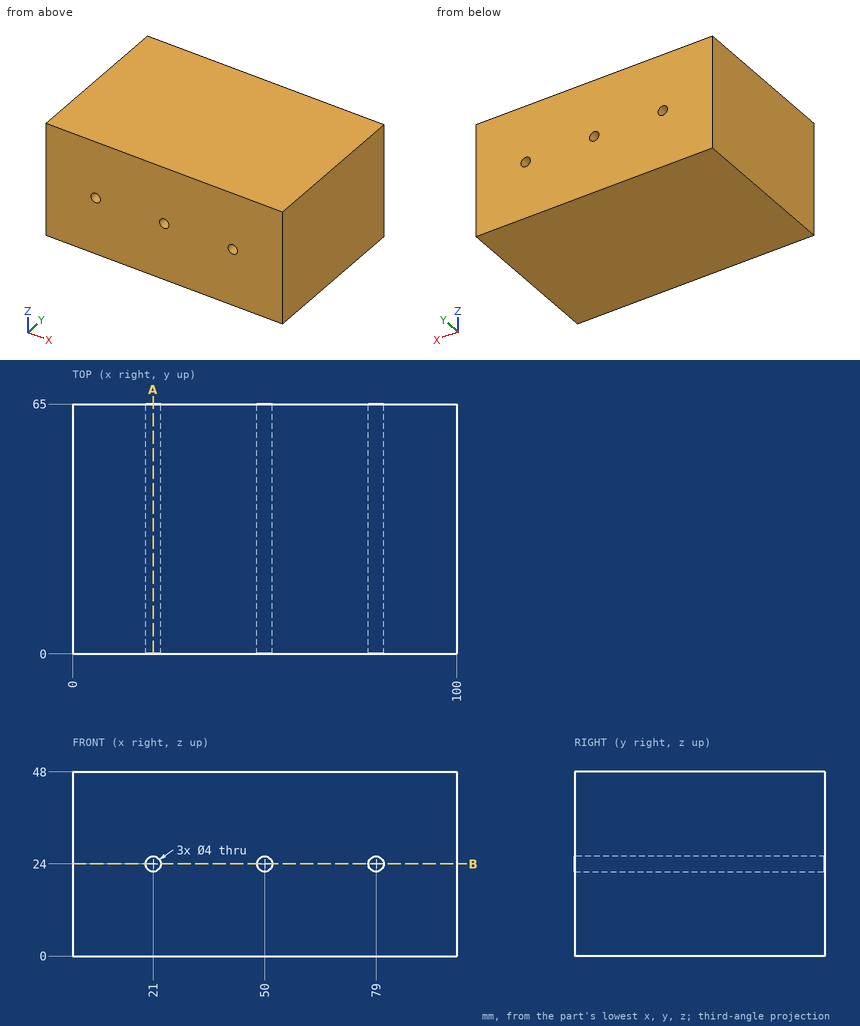
Check sheet for the drawn part. Datum: minimum x, y, z corner. Units: mm. Round coordinates to 2 decimals unless told otherwise and drop trailing zeros. Write each loop counter-clockwise with the first axis right and the second up, starting at its lowest first coordinate (ties: lowest second). Pieces come first, ordered by that corner, then holes. Notation, with made-up numbers: (7, 74.5) -> (61, 74.5) arc R19 ccw to (61, 101.5) -> close; hole circle Ø1 at (89, 67.25). An arc over 180 degrees is marked (long way). Write each question's results on one line, items separated by ' | '. Start each with the question number.
1. Cross-section at A-A (x = 21). Enter the section's corners in (y, z).
2. Depth check by flat-ended pin: P1, Ø10, axis at x = 60, y = 7, coming from the -Z side. Enter the tip coordinate at first touch or a pass-through.
3. Material ranges on probe 1 along X at (y, z) = (30, 24); probe 2 along Z at (x, y) = (79, 47); probe 3 along Z at (x, y) = (20.5, 59.5), recorded low to high. Write a range as from..to.
4. Cross-section at B-B (z = 24). Enter the section's corners in (x, y), then the cut area to 3 significant figures.
Solutions:
1) outline: (0, 0) -> (65, 0) -> (65, 22) -> (0, 22) -> close; (0, 26) -> (65, 26) -> (65, 48) -> (0, 48) -> close
2) P1: stops at z = 0
3) probe 1: x = 0..19, 23..48, 52..77, 81..100 | probe 2: z = 0..22, 26..48 | probe 3: z = 0..22.06, 25.94..48
4) outline: (0, 0) -> (19, 0) -> (19, 65) -> (0, 65) -> close; (23, 0) -> (48, 0) -> (48, 65) -> (23, 65) -> close; (52, 0) -> (77, 0) -> (77, 65) -> (52, 65) -> close; (81, 0) -> (100, 0) -> (100, 65) -> (81, 65) -> close | area: 5,720 mm2
